Build history of the part. All positions in model axes, mm. A direction names the side the tool comes from. Give positions to 0.01 mm unless a question says otherwise; leave off trailing zeros. Order: outer loops, then holes, each group sorted by start corner. A loop starts at its lowest first (then second) coordinate and runs counter-clockwise, first axis right, second up. Notation, with made-up numbers: M -34,45.5 L -1,45.5 A27 ccw -1,84.5 Z; hole C 13,-40 d10. An arc over 180 degrees is marked long. Use CSV: the item, a comma, the result in double quotes. Start each with the question number.
Item 1: Pin check, flat tips, straight feed: P1, Ø3, axis at y = 46.5, z = 19.5, coming from the +X side; P2, Ø14, axis at x = 61, y = 4, coming from the -Z side; P3, Ø3.5, axis at x = -58, z = 21.5, coming from the +Y side; P4, Ø2.5, axis at x = 58.36, y = 0, coming from the -Z side. Stop position of each tip, or through.
Item 2: Wall check: line 1 along Z through (x, y) = (-7, -11); line 2 along Y through (x, z) = (-57, 22.25); line 3 along X through (y, z) = (26.5, 15.5). Give the ranges that are in metal, low to high.
Item 3: Two-plate mould, pull along X, no slides. Class faces 1 (the flat face through (-1, 1, 2)), 2 (the flat face through (58, -5.488, 23)), 3 (the cylindrical face through (53.301, -6.675, 22.465)): pulls with the +X half, pulls with the -X half, needs draft (parallel to the pull), parting line crosses it, or undercut.
Item 4: Which spindle directions (+Z, -Z, +X, -X, +Y, -Y) get a long thin tool onto all of the face, cutting with end or side? Do faces 4 (the cylindrical face through (63.012, 4.062, 22.465)), 5 (the flat face through (-58, -5.488, 23)), 6 (the flat face through (8, 48, 19)), 7 (the flat face through (-58, 5.488, 23)), 8 (the conical face through (-8.999, -40.526, 0.971)). Say none if no direction does.
Item 5: Band-saw the part on B-B on z = 10. Write the cut outline in (x, y), plus the area to 3 significant figures.
Item 6: Band-saw the part on A-A on x = 0. Write the cut outline in (y, z), plus the area to 3 significant figures.
from build123d import *

# Parameters (mm, degrees)
F0_R        = 52.5
F0_R_2      = 49
F1_DEPTH    = 2
F2_DEPTH    = 25
F3_SIZE2    = 11.5470053838
F3_SIZE     = 20
F4_SIZE2    = 11.5470053838
F4_SIZE     = 20
F6_DEPTH    = 13
F7_R        = 2.25
F8_DEPTH    = 5
F9_T1_DEPTH = 5
F9_T3_DEPTH = 5


# Not quite as in the source:
# - a fillet or chamfer that OpenCascade refuses, or shapes differently, is made with other operations: its cross-section is extruded or revolved along the edge and cut away or added


with BuildPart() as f1:
    # F0 (on Top) → F1 (new body)
    with BuildSketch(Plane.XY):
        Circle(F0_R)
        Circle(F0_R_2, mode=Mode.SUBTRACT)
        Circle(F0_R_2)
    extrude(amount=F1_DEPTH)

    # F0 (on Top) → F2 (join)
    with BuildSketch(Plane.XY):
        Circle(F0_R)
        Circle(F0_R_2, mode=Mode.SUBTRACT)
    extrude(amount=F2_DEPTH)

    # F3
    f3_edges = [f1.edges().sort_by_distance(p)[0] for p in [
        (-49, 0, 2),
    ]]
    chamfer(f3_edges, length=F3_SIZE, length2=F3_SIZE2)

    # F4
    f4_edges = [f1.edges().sort_by_distance(p)[0] for p in [
        (-52.5, 0, 0),
    ]]
    f4_side = f1.faces().sort_by_distance((-52.5, 0, 12.5))[0]
    chamfer(f4_edges, length=F4_SIZE, length2=F4_SIZE2, reference=f4_side)

    # F5 (on face) → F6 (cut)
    with BuildSketch(Plane.XY.offset(25)):
        with BuildLine():
            Line((8, 51.8868962263), (8, 67.5))
            Line((8, 67.5), (-8, 67.5))
            Line((-8, 67.5), (-8, 51.8868962263))
            ThreePointArc((-8, 51.8868962263), (0, 52.5), (8, 51.8868962263))
        make_face()
        with BuildLine():
            Line((8, 48.3425278611), (8, 51.8868962263))
            ThreePointArc((8, 51.8868962263), (0, 52.5), (-8, 51.8868962263))
            Line((-8, 51.8868962263), (-8, 48.3425278611))
            ThreePointArc((-8, 48.3425278611), (0, 49), (8, 48.3425278611))
        make_face()
        with BuildLine():
            Line((8, 37.5), (8, 48.3425278611))
            ThreePointArc((8, 48.3425278611), (0, 49), (-8, 48.3425278611))
            Line((-8, 48.3425278611), (-8, 37.5))
            Line((-8, 37.5), (8, 37.5))
        make_face()
    extrude(amount=-F6_DEPTH, mode=Mode.SUBTRACT)

    # F7 (on face) → F8 (join)
    with BuildSketch(Plane.XY.offset(25)):
        with BuildLine():
            Line((-64.5158270159, -5.4877443216), (-52.2123995068, -5.4877443216))
            ThreePointArc((-52.2123995068, -5.4877443216), (-52.5, 0), (-52.2123995068, 5.4877443216))
            Line((-52.2123995068, 5.4877443216), (-64.5158270159, 5.4877443216))
            Line((-64.5158270159, 5.4877443216), (-64.5158270159, -5.4877443216))
        make_face()
        with Locations((-58.3641132614, 0)):
            Circle(F7_R, mode=Mode.SUBTRACT)
        with BuildLine():
            ThreePointArc((52.2123995068, 5.4877443216), (52.5, 0), (52.2123995068, -5.4877443216))
            Line((52.2123995068, -5.4877443216), (64.5158270159, -5.4877443216))
            Line((64.5158270159, -5.4877443216), (64.5158270159, 5.4877443216))
            Line((64.5158270159, 5.4877443216), (52.2123995068, 5.4877443216))
        make_face()
        with Locations((58.3641132614, 0)):
            Circle(F7_R, mode=Mode.SUBTRACT)
    extrude(amount=-F8_DEPTH)

    # F9: fillet of radius 5 on 8 edges, made by hand

    # F9_s2 → F9_t1 (join)
    with BuildSketch(Plane.XY.offset(20)):
        with BuildLine():
            ThreePointArc((-51.6193248202, -9.5757665545), (-53.3385688277, -6.6432749931), (-56.5354509936, -5.4877443216))
            Line((-56.5354509936, -5.4877443216), (-56.5354509936, -5.3877443216))
            Line((-56.5354509936, -5.3877443216), (-52.2123995068, -5.3877443216))
            Line((-52.2123995068, -5.3877443216), (-52.1129473173, -5.4772914752))
            ThreePointArc((-52.1129473173, -5.4772914752), (-51.8571206165, -7.5232334382), (-51.5210022967, -9.5575269991))
            Line((-51.5210022967, -9.5575269991), (-51.6193248202, -9.5757665545))
        make_face()
        with BuildLine():
            ThreePointArc((-51.6193248202, 9.5757665545), (-53.3385688277, 6.6432749931), (-56.5354509936, 5.4877443216))
            Line((-56.5354509936, 5.4877443216), (-56.5354509936, 5.3877443216))
            Line((-56.5354509936, 5.3877443216), (-52.2123995068, 5.3877443216))
            Line((-52.2123995068, 5.3877443216), (-52.1129473173, 5.4772914752))
            ThreePointArc((-52.1129473173, 5.4772914752), (-51.8571206165, 7.5232334382), (-51.5210022967, 9.5575269991))
            Line((-51.5210022967, 9.5575269991), (-51.6193248202, 9.5757665545))
        make_face()
        with BuildLine():
            ThreePointArc((51.6193248202, -9.5757665545), (53.3385688277, -6.6432749931), (56.5354509936, -5.4877443216))
            Line((56.5354509936, -5.4877443216), (56.5354509936, -5.3877443216))
            Line((56.5354509936, -5.3877443216), (52.2123995068, -5.3877443216))
            Line((52.2123995068, -5.3877443216), (52.1129473173, -5.4772914752))
            ThreePointArc((52.1129473173, -5.4772914752), (51.8571206165, -7.5232334382), (51.5210022967, -9.5575269991))
            Line((51.5210022967, -9.5575269991), (51.6193248202, -9.5757665545))
        make_face()
        with BuildLine():
            ThreePointArc((51.6193248202, 9.5757665545), (53.3385688277, 6.6432749931), (56.5354509936, 5.4877443216))
            Line((56.5354509936, 5.4877443216), (56.5354509936, 5.3877443216))
            Line((56.5354509936, 5.3877443216), (52.2123995068, 5.3877443216))
            Line((52.2123995068, 5.3877443216), (52.1129473173, 5.4772914752))
            ThreePointArc((52.1129473173, 5.4772914752), (51.8571206165, 7.5232334382), (51.5210022967, 9.5575269991))
            Line((51.5210022967, 9.5575269991), (51.6193248202, 9.5757665545))
        make_face()
    extrude(amount=F9_T1_DEPTH)

    # F9_s4 → F9_t3 (cut)
    with BuildSketch(Plane.XY.offset(20)):
        with BuildLine():
            ThreePointArc((-59.5158270159, -5.4877443216), (-63.0513609218, -4.0232782275), (-64.5158270159, -0.4877443216))
            Line((-64.5158270159, -0.4877443216), (-64.6158270159, -0.4877443216))
            Line((-64.6158270159, -0.4877443216), (-64.6158270159, -5.5877443216))
            Line((-64.6158270159, -5.5877443216), (-59.5158270159, -5.5877443216))
            Line((-59.5158270159, -5.5877443216), (-59.5158270159, -5.4877443216))
        make_face()
        with BuildLine():
            ThreePointArc((-64.5158270159, 0.4877443216), (-63.0513609218, 4.0232782275), (-59.5158270159, 5.4877443216))
            Line((-59.5158270159, 5.4877443216), (-59.5158270159, 5.5877443216))
            Line((-59.5158270159, 5.5877443216), (-64.6158270159, 5.5877443216))
            Line((-64.6158270159, 5.5877443216), (-64.6158270159, 0.4877443216))
            Line((-64.6158270159, 0.4877443216), (-64.5158270159, 0.4877443216))
        make_face()
        with BuildLine():
            ThreePointArc((64.5158270159, -0.4877443216), (63.0513609218, -4.0232782275), (59.5158270159, -5.4877443216))
            Line((59.5158270159, -5.4877443216), (59.5158270159, -5.5877443216))
            Line((59.5158270159, -5.5877443216), (64.6158270159, -5.5877443216))
            Line((64.6158270159, -5.5877443216), (64.6158270159, -0.4877443216))
            Line((64.6158270159, -0.4877443216), (64.5158270159, -0.4877443216))
        make_face()
        with BuildLine():
            ThreePointArc((59.5158270159, 5.4877443216), (63.0513609218, 4.0232782275), (64.5158270159, 0.4877443216))
            Line((64.5158270159, 0.4877443216), (64.6158270159, 0.4877443216))
            Line((64.6158270159, 0.4877443216), (64.6158270159, 5.5877443216))
            Line((64.6158270159, 5.5877443216), (59.5158270159, 5.5877443216))
            Line((59.5158270159, 5.5877443216), (59.5158270159, 5.4877443216))
        make_face()
    extrude(amount=F9_T3_DEPTH, mode=Mode.SUBTRACT)


solid = f1.part
Model answer:
1,P1,"stops at x = 26.9"
1,P2,"stops at z = 20"
1,P3,"stops at y = 5.5"
1,P4,"passes through"
2,line 1,"z = 0 to 2"
2,line 2,"y = -5.49 to -1.79, 1.79 to 5.49"
2,line 3,"x = -42.28 to -36.68, 36.68 to 42.28"
3,face 1,"undercut"
3,face 2,"needs draft"
3,face 3,"pulls with the +X half"
4,face 4,"+Z, -Z, +X, +Y"
4,face 5,"+Z, -Z, -X, -Y"
4,face 6,"+Z, +Y"
4,face 7,"+Z, -Z, -X, +Y"
4,face 8,"-Z"
5,outline,"C 0,0 d93.45; hole C 0,0 d84.14"
5,area,"1,300 mm^2"
6,outline,"M -52.5,20 L -40.95,0 L 40.95,0 L 47.88,12 L 43.23,12 L 37.45,2 L -37.45,2 L -49,22 L -49,25 L -52.5,25 Z"
6,area,"315 mm^2"
